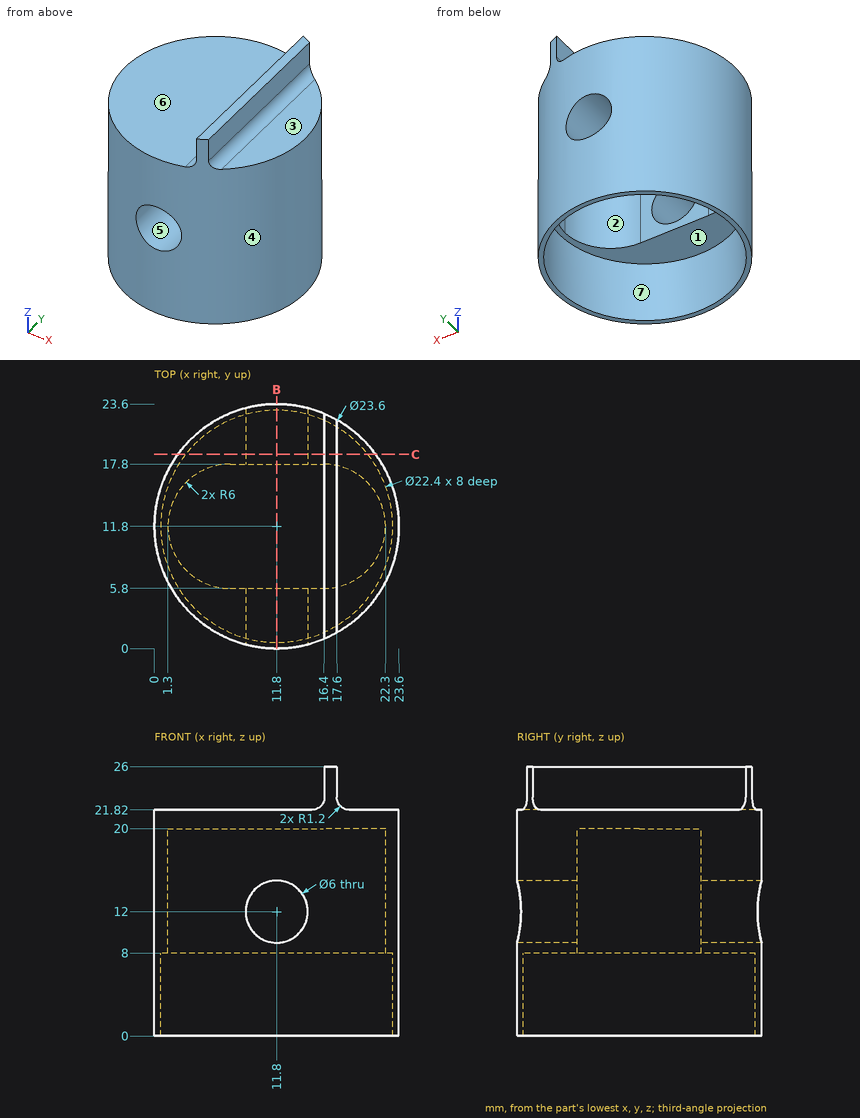
Input: dimensioned drawing with shaded views. Units: mm. Origin: part minimum x, y, z. A direction names the side the tool comes from. Give positions to 0.01 mm unless a question says otherwise; leave off trailing zeros. Loops run counter-clockwise (first coordinate to the right, second up) from the corner with the lowest first, then second, coordinate; pieces in that order, holes last. Notation, with made-up numbers: (10, 81) -> (20, 81) arc R34 ccw to (20, 116) -> close; hole circle Ø1 at (74.25, 69). An arc over 180 degrees is marked (long way). Use a Markdown table: item, result. Add a question column.
1) Line query: line 1 along Z through (x, y) = (11.8, 20.85); line 2 along Y through (x, z) = (11.8, 6); line 3 along Z through (x, y) = (14.5, 10.5). Output: solid intervals per line, ascending. Write a range as [from, to].
2) Pull-direction query (Y, two-part tool) for the marked faces 1, 2, 3 and 4; classes: +Y half, -Y half, draft (parallel to the pull), parting line (faces both ways), or undercut.
3) Section query C-C, the plane y = 18.75. Return the cut outline in (x, z), then the cut area to 3 significant figures.
4) Reachability of the marked faces 5, 6 and 7 from +Z, -Z, +X, -X, +Y, -Y: full face, straight path, thin tool, end or side. Return the list, or none.
5) First-contact query: pin 1 (2.5 mm diameter, centred on y = 14.5, z = 24.5, fed in from +X); pin 2 (3 mm diameter, centred on y = 8, z = 14.5, fed in from -X); pin 3 (5 mm diameter, centred on x = 11.8, z = 12, fed in from -Y); pin 4 (3.5 mm diameter, centred on x = 12.5, y = 14.5, fed in from -Z). Flat tips, straight axial feed; report the tip coordinate or a pass-through.
6) Section query B-B, the plane x = 11.8. Return the cut outline in (y, z).
Numbers:
| question | item | result |
|---|---|---|
| 1 | line 1 | z = [8, 9], [15, 21.82] |
| 1 | line 2 | y = [0, 0.6], [23, 23.6] |
| 1 | line 3 | z = [20, 21.82] |
| 2 | face 1 | undercut |
| 2 | face 2 | undercut |
| 2 | face 3 | draft |
| 2 | face 4 | parting line |
| 3 | outline | (2.26, 0) -> (3.02, 0) -> (3.02, 8) -> (20.58, 8) -> (20.58, 0) -> (21.34, 0) -> (21.34, 21.82) -> (18.8, 21.82) arc R1.2 cw to (17.6, 23.02) -> (17.6, 26) -> (16.4, 26) -> (16.4, 23.02) arc R1.2 cw to (15.2, 21.82) -> (2.26, 21.82) -> close; hole circle Ø6 at (11.8, 12) |
| 3 | area | 253 mm2 |
| 4 | face 5 | +Y, -Y |
| 4 | face 6 | +Z, -X, +Y, -Y |
| 4 | face 7 | -Z |
| 5 | pin 1 | stops at x = 17.6 |
| 5 | pin 2 | stops at x = 0.23 |
| 5 | pin 3 | passes through |
| 5 | pin 4 | stops at z = 20 |
| 6 | outline | (0, 0) -> (0.6, 0) -> (0.6, 8) -> (5.8, 8) -> (5.8, 9) -> (0, 9) -> close; (0, 15) -> (5.8, 15) -> (5.8, 20) -> (17.8, 20) -> (17.8, 15) -> (23.6, 15) -> (23.6, 21.82) -> (0, 21.82) -> close; (17.8, 8) -> (23, 8) -> (23, 0) -> (23.6, 0) -> (23.6, 9) -> (17.8, 9) -> close |
